```python
from build123d import *

# Parameters (mm, degrees)
F0_R     = 21.4542850261
F1_DEPTH = 65.786
F2_R     = 5.08
F3_T     = -2.54


# Not quite as in the source:
# - a shell that OpenCascade refuses in one call is made with other operations: the cavity is built on its own and cut out


with BuildPart() as f1:
    # F0 (on Top) → F1 (new body)
    with BuildSketch(Plane.XY):
        with Locations((-44.2928858101, 29.3457191437)):
            Circle(F0_R)
    extrude(amount=F1_DEPTH)

    # F2
    f2_edges = [f1.edges().sort_by_distance(p)[0] for p in [
        (-65.747171, 29.345719, 65.786),
    ]]
    fillet(f2_edges, radius=F2_R)

    # F3: a shell. OpenCascade refuses it in one call, so the cavity is built on its own and cut out:
    # the body offset inwards by the wall thickness, plus a prism from it out through each open face.
    f3_core = offset(f1.part, amount=F3_T, mode=Mode.PRIVATE)
    f3_exits = [f3_core.faces().sort_by_distance(p)[0] for p in [
        (-44.292886, 29.345719, 63.246),
    ]]
    add(f3_core, mode=Mode.SUBTRACT)
    extrude(f3_exits, amount=-F3_T, mode=Mode.SUBTRACT)


solid = f1.part
```
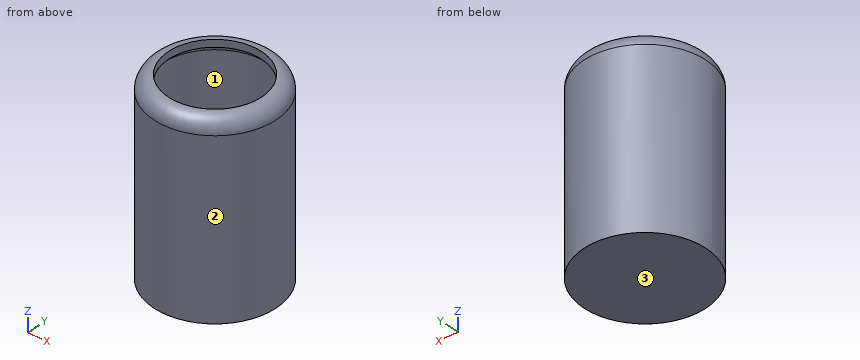
Check sheet for the modelled part. Datum: model origin and axes. Units: mm. Face numbers are marked on the shaded views. Coordinates: 2 decimals unless noted, no trailing zeros. Order: outer loops, then holes, each group sorted by start corner. A loop starts at its lowest first (then second) coordinate and runs counter-clockwise, first axis right, second up. Notation, with made-up numbers: (-4.5, 77.5) -> (34.5, 77.5) arc R22 cw to (34.5, 96.5) -> close; hole circle Ø5 at (27, -27.5). An arc over 180 degrees is marked (long way). Write item = value, one per line. Start each with the question number.
1) Material ranges on L1, parallel to X at y = 29, z = 30; L2, parallel to Z at x = -36, y = 43; L3, parallel to Z at x = -31.5, y = 17, recorded low to high.
2) Go/stop test with flat-tipped pins: P1, Ø1, axis at x = -59.5, z = 21, coming from the +Y side; P2, Ø2, axis at x = -52.5, z = 18.5, coming from the -Y side; P3, Ø5, axis at x = -40, y = 19.5, coming from the +Z side. Record where each tip stops, or that it passes through.
3) Mould release check, pull along Z, two halves, no side actions. Record for the marked faces 1, 2 and 3: +Z half, -Z half, draft (parallel to the pull), parting line (faces both ways), or undercut.
4) Cross-section at A-A (z = 23.5). Enter the section's corners in (x, y), then the cut area to 3 significant figures.
Ans:
q1.L1 = -65.74 to -63.2, -25.38 to -22.84
q1.L2 = 0 to 2.54
q1.L3 = 0 to 2.54, 62.82 to 65.59
q2.P1 = 44.97
q2.P2 = 9.14
q2.P3 = 2.54
q3.face_1 = undercut
q3.face_2 = draft
q3.face_3 = -Z half
q4.outline = circle Ø42.91 at (-44.29, 29.35); hole circle Ø37.83 at (-44.29, 29.35)
q4.area = 322 mm²
